Can you work these out from the model? Positions are in its coordinate system, mm. A direction names the side the tool comes from. Give positions to 0.01 mm unless a question says otherwise; leave off trailing zeros. Order: outer loops, then holes, each group sorted by start corner. A loop starts at its lowest first (then second) coordinate and runs counter-clockwise, first axis right, second up. Notation, with made-up numbers: M -22,36.25 L -6,36.25 A34 ccw -6,73.25 Z; hole C 1.5,26 d5. An arc over 180 degrees is marked long. Answer as a JSON object with one key per item and string values.
Autodesk Inventor part; units mm, degrees
ref_plane "YZ Plane" through (0, 0, 0) normal (1, 0, 0) x (0, 1, 0)
ref_plane "XZ Plane" through (0, 0, 0) normal (0, 1, 0) x (-1, 0, 0)
ref_plane "XY Plane" through (0, 0, 0) normal (0, 0, 1) x (1, 0, 0)
sketch "Sketch1" plane through (0, 0, 0) normal (0, 1, 0) x (-1, 0, 0)
  circle A0 centre (0, 0) radius 9.0297
  dimension "d0" = 18.0594
extrude "Extrusion1" add sketch "Sketch1" along normal blind 21.082
sketch "Sketch2" plane through (0, 21.082, 0) normal (0, 1, 0) x (1, 0, 0)
  circle A0 centre (0, 0) radius 4.9276
  circle A1 centre (0, 0) radius 9.0297
  dimension "d3" = 9.8552
  dimension "d4" = 18.0594
extrude "Extrusion2" cut sketch "Sketch2" against normal blind 4.9784
sketch "Sketch3" plane through (0, 0, 0) normal (0, -1, 0) x (1, 0, 0)
  circle A0 centre (0, 0) radius 3.1306
  dimension "d7" = 6.2611
extrude "Extrusion3" cut sketch "Sketch3" against normal blind 203.2
properties part number "Wire fitting End"
1) I want a section at B-B on z = 0. Write out the boundary of the cut face in (x, y), and give its area (3 significant figures).
Results found:
{"outline": "M -9.03,0 L -3.13,0 L -3.13,21.08 L -4.93,21.08 L -4.93,16.1 L -9.03,16.1 Z; M 3.13,0 L 9.03,0 L 9.03,16.1 L 4.93,16.1 L 4.93,21.08 L 3.13,21.08 Z", "area": "208 mm²"}
2) I need wall thicknesses on L1, parallel to Z at x = 0, y = 7; L2, parallel to Y at x = -5.75, z = 0.75; L3, parallel to Z at x = 0, y = 16.25. Which ranges of each line are inside material? Lowest first, please.
Results found:
{"L1": "z = -9.03 to -3.13, 3.13 to 9.03", "L2": "y = 0 to 16.1", "L3": "z = -4.93 to -3.13, 3.13 to 4.93"}
3) For faces 4 (the face through (4, 16.104, 4)), 5 (the face through (-1, 21.082, -3.2)), which set-ups out of +Z, -Z, +X, -X, +Y, -Y let a thin tool reach every point of the face, with its end or its side?
Results found:
{"face 4": "+Y", "face 5": "+Z, -Z, +X, -X, +Y"}
4) Thinking about a two-plate mould opening in X: for faces 1 (the face through (-4, 0, 0)), 2 (the face through (3, 10.4, 0.9)), 3 (the face through (1.175, 7.939, -8.953)), which applies, pulls with the +X half, pulls with the -X half, needs draft (parallel to the pull), parting line crosses it, or undercut?
Results found:
{"face 1": "needs draft", "face 2": "undercut", "face 3": "parting line crosses it"}
5) I want a section at A-A on x = 0. Write out the boundary of the cut face in (y, z).
Results found:
{"outline": "M 0,-9.03 L 16.1,-9.03 L 16.1,-4.93 L 21.08,-4.93 L 21.08,-3.13 L 0,-3.13 Z; M 0,3.13 L 21.08,3.13 L 21.08,4.93 L 16.1,4.93 L 16.1,9.03 L 0,9.03 Z"}
6) I want a section at D-D on x = -4.5. Write out the boundary of the cut face in (y, z).
Results found:
{"outline": "M 0,-7.83 L 16.1,-7.83 L 16.1,-2.01 L 21.08,-2.01 L 21.08,2.01 L 16.1,2.01 L 16.1,7.83 L 0,7.83 Z"}
7) I want a section at C-C on y = 2.75. Write out the boundary of the cut face in (x, z), and give its area (3 significant figures).
Results found:
{"outline": "C 0,0 d18.06; hole C 0,0 d6.26", "area": "225 mm²"}
8) I'm going to push flat-ended pins straight in: pin 1 Ø1.5 at (x, y) = (1, 7.5) entering from -Z; pin 2 Ø1 at (x, z) = (4.5, -6.5) entering from -Y; pin 3 Ø1.5 at (x, y) = (-6, 8.5) entering from -Z. Where does each tip first touch, or does it pass through?
Results found:
{"pin 1": "stops at z = -9.03", "pin 2": "stops at y = 0", "pin 3": "stops at z = -7.35"}
